from build123d import *

# Parameters (mm, degrees)
SALIENTE_EXTRUIR3_DEPTH = 2
SALIENTE_EXTRUIR4_START = -2
CROQUIS3_R              = 2
SALIENTE_EXTRUIR4_DEPTH = 3


with BuildPart() as part:
    # Croquis1 → Saliente-Extruir3 (new body)
    with BuildSketch(Plane(origin=(0, 0, 0), x_dir=(1, 0, 0), z_dir=(0, 1, 0))):
        Polygon((-17.5, 5), (-17.5, -5), (-17.5, -15), (17.5, -15), (17.5, -6), (17.5, -4), (12.5, -4), (12.5, -6), (-9, -6), (-9, 8.019718755), (6.986881597, 8.019718755), (6.986881597, 10), (17.5, 10), (17.5, 15), (5, 15), (-5, 15), (-17.5, 15), align=None)
    extrude(amount=SALIENTE_EXTRUIR3_DEPTH)

    # Croquis3 → Saliente-Extruir4 (add)
    # profile 1 of 2: a face of its own
    with BuildSketch(Plane(origin=(0, 0, -15), x_dir=(-1, 0, 0), z_dir=(0, 0, -1)).offset(SALIENTE_EXTRUIR4_START)):
        with BuildLine():
            Line((-17.5, 2), (-17.5, -6))
            Line((-17.5, -6), (-22.5, -6))
            ThreePointArc((-22.5, -6), (-26.5, -2), (-22.5, 2))
            Line((-22.5, 2), (-17.5, 2))
        make_face()
        with Locations((-22.5, -2)):
            Circle(CROQUIS3_R, mode=Mode.SUBTRACT)
    # profile 2 of 2: a face of its own
    with BuildSketch(Plane(origin=(0, 0, -15), x_dir=(-1, 0, 0), z_dir=(0, 0, -1)).offset(SALIENTE_EXTRUIR4_START)):
        with BuildLine():
            Line((17.5, 2), (17.5, -6))
            Line((17.5, -6), (22.5, -6))
            ThreePointArc((22.5, -6), (26.5, -2), (22.5, 2))
            Line((22.5, 2), (17.5, 2))
        make_face()
        with Locations((22.5, -2)):
            Circle(CROQUIS3_R, mode=Mode.SUBTRACT)
    extrude(amount=-SALIENTE_EXTRUIR4_DEPTH)


solid = part.part
Check sheet for the modelled part. Datum: model origin and axes. Units: mm. A direction names the side the tool comes from. Round coordinates to 2 decimals unless told otherwise and drop trailing zeros. Write each loop counter-clockwise with the first axis right and the second up, starting at its lowest first coordinate (ties: lowest second). Pieces come first, ordered by that corner, then holes. Notation, with made-up numbers: (16.25, 6.25) -> (43.25, 6.25) arc R10 cw to (43.25, 11.25) -> close; hole circle Ø5 at (14, 68). An arc over 180 degrees is marked (long way). Answer as CSV lines item,"result". Start each with the question number.
1) Material ranges on line 1 (X direction, y = -3.5, z = -10.5); line 2 (Y direction, x = 10.5, z = -11); line 3 (Z direction, x = -22.5, y = -5.5), recorded low to high. Write a range as from..to.
2) Go/stop test with flat-tipped pins: P1, Ø2, axis at y = 0.5, z = -1.5, coming from the +X side; P2, Ø0.9, axis at y = -4, z = -12, coming from the +X side; P3, Ø8, axis at x = -8.5, z = -2.5, coming from the -Y side. Record where each tip stops, or that it passes through.
3) Tool access check on faces 4 (the flat face through (-20, -2, -13)), 5 (the flat face through (17.5, 1, -14)), 6 (the flat face through (17.5, -3, -12)). Record the directions out of +Z, -Z, +X, -X, +Y, -Y that give a thin tool (end or side, any length) a straight path to the whole face; none if there is none.
4) Release check for a two-part mould opening along X. For faces 1 (the cylindrical face through (24.1, -3.2, -11.5)), 2 (the flat face through (-17.5, 1, 2)), 3 (the flat face through (17.5, 1, 10)) record: pulls with the +X half, pulls with the -X half, needs draft (parallel to the pull), parting line crosses it, or undercut.
5) Section check D-D on x = -18. Enter the section's corners in (y, z).
6) Section check B-B on x = 0.5. Enter the section's corners in (y, z), and give its area (3 significant figures).
7) Section check C-C on z = -11.75. Enter the section's corners in (x, y), and give its area (3 significant figures).
8) Section check A-A on y = -2. Enter the section's corners in (x, z), and give its area (3 significant figures).
Found:
1,line 1,"x = -26.21..-23.82, -21.18..-17.5, 17.5..21.18, 23.82..26.21"
1,line 2,"y = 0..2"
1,line 3,"z = -13..-10"
2,P1,"stops at x = -9"
2,P2,"stops at x = 26.19"
2,P3,"stops at y = 0"
3,face 4,"-Z, -X, +Y, -Y"
3,face 5,"-Z, +X, +Y, -Y"
3,face 6,"+Z, -Z, -Y"
4,face 1,"undercut"
4,face 2,"pulls with the -X half"
4,face 3,"pulls with the +X half"
5,outline,"(-6, -13) -> (2, -13) -> (2, -10) -> (-6, -10) -> close"
6,outline,"(0, -15) -> (2, -15) -> (2, -8.02) -> (0, -8.02) -> close; (0, 6) -> (2, 6) -> (2, 15) -> (0, 15) -> close"
6,area,"32.0 mm^2"
7,outline,"(-22.5, -6) -> (-17.5, -6) -> (-17.5, 0) -> (17.5, 0) -> (17.5, -6) -> (22.5, -6) arc R4 ccw to (22.5, 2) -> (-22.5, 2) arc R4 ccw to start; hole circle Ø4 at (-22.5, -2); hole circle Ø4 at (22.5, -2)"
7,area,"175 mm^2"
8,outline,"(-26.5, -13) -> (-24.5, -13) -> (-24.5, -10) -> (-26.5, -10) -> close; (-20.5, -13) -> (-17.5, -13) -> (-17.5, -10) -> (-20.5, -10) -> close; (17.5, -13) -> (20.5, -13) -> (20.5, -10) -> (17.5, -10) -> close; (24.5, -13) -> (26.5, -13) -> (26.5, -10) -> (24.5, -10) -> close"
8,area,"30.0 mm^2"
